```python
from build123d import *

# Parameters (mm, degrees)
F0_R     = 5.3
F0_R_2   = 4.1
F1_DEPTH = 4
F2_SIZE  = 0.5
F3_R     = 0.5


with BuildPart() as f1:
    # F0 (on Top) → F1 (new body)
    with BuildSketch(Plane.XY):
        Circle(F0_R)
        Circle(F0_R_2, mode=Mode.SUBTRACT)
    extrude(amount=F1_DEPTH)

    # F2
    f2_edges = [f1.edges().sort_by_distance(p)[0] for p in [
        (-4.1, 0, 0),
    ]]
    chamfer(f2_edges, length=F2_SIZE)

    # F3
    f3_edges = [f1.edges().sort_by_distance(p)[0] for p in [
        (-5.3, 0, 4),
    ]]
    fillet(f3_edges, radius=F3_R)


solid = f1.part
```
CAD build for the part. Positions are in the model's coordinates, mm. Round coordinates to 2 decimals unless told otherwise and drop trailing zeros. Order: outer loops, then holes, each group sorted by start corner. A loop starts at its lowest first (then second) coordinate and runs counter-clockwise, first axis right, second up.
Q1. Slice it at C-C (z = 2.85). Write the cut outline in (x, y), and give its area (3 significant figures).
Q2. Wall check: L1, parallel to Y at x = 0, z = 2.4; L2, parallel to X at y = -1.25, z = 2.55; L3, parallel to X at y = -0.5, z = 3.1. Give the ranges that are in metal, low to high.
Q3. Slice it at A-A (x = 0). Write the cut outline in (y, z).
Q4. Drop flat-ended pins along their axis: pin 1 (2 mm diameter, centred on y = -3.5, z = 2.5, fed in from +X); pin 2 (2 mm diameter, centred on x = 2.5, z = 1.5, fed in from +Y). Give the stop position or say it passes through.
Q5. Slice it at D-D (z = 3.65). Write the cut outline in (x, y).
Q6. Two-plate mould, pull along Y, no slides. Class faces 1 (the cylindrical face through (4.896, -2.03, 1.726)), 2 (the flat face through (4, 2, 4)), 3 (the cylindrical face through (-0.534, 4.065, 2.226)): pulls with the +Y half, pulls with the -Y half, needs draft (parallel to the pull), parting line crosses it, or undercut.
Results below:
1. outline: circle Ø10.6 at (0, 0); hole circle Ø8.2 at (0, 0)
1. area: 35.4 mm2
2. L1: y = -5.3 to -4.1, 4.1 to 5.3
2. L2: x = -5.15 to -3.9, 3.9 to 5.15
2. L3: x = -5.28 to -4.07, 4.07 to 5.28
3. outline: (-5.3, 0) - (-4.6, 0) - (-4.1, 0.5) - (-4.1, 4) - (-4.8, 4) arc R0.5 ccw to (-5.3, 3.5) - close; (4.1, 0.5) - (4.6, 0) - (5.3, 0) - (5.3, 3.5) arc R0.5 ccw to (4.8, 4) - (4.1, 4) - close
4. pin 1: stops at x = 4.67
4. pin 2: stops at y = 5.08
5. outline: circle Ø10.55 at (0, 0); hole circle Ø8.2 at (0, 0)
6. face 1: parting line crosses it
6. face 2: needs draft
6. face 3: undercut
